Could you check a few things on this drawing? It's one solid part, dimensions in mm from its lowest x, y, z. Round coordinates to 2 decimals unless told otherwise and drop trailing zeros. Loops run counter-clockwise (first coordinate to the right, second up) from the corner with the lowest first, then second, coordinate; pieces in that order, holes last. Notation, with made-up numbers: M -8,14 L 12,14 A13 cw 12,29 Z; hole C -20.75,-32.5 d11. An arc over 180 degrees is marked long. Return JSON: item names as keys, results as strings.
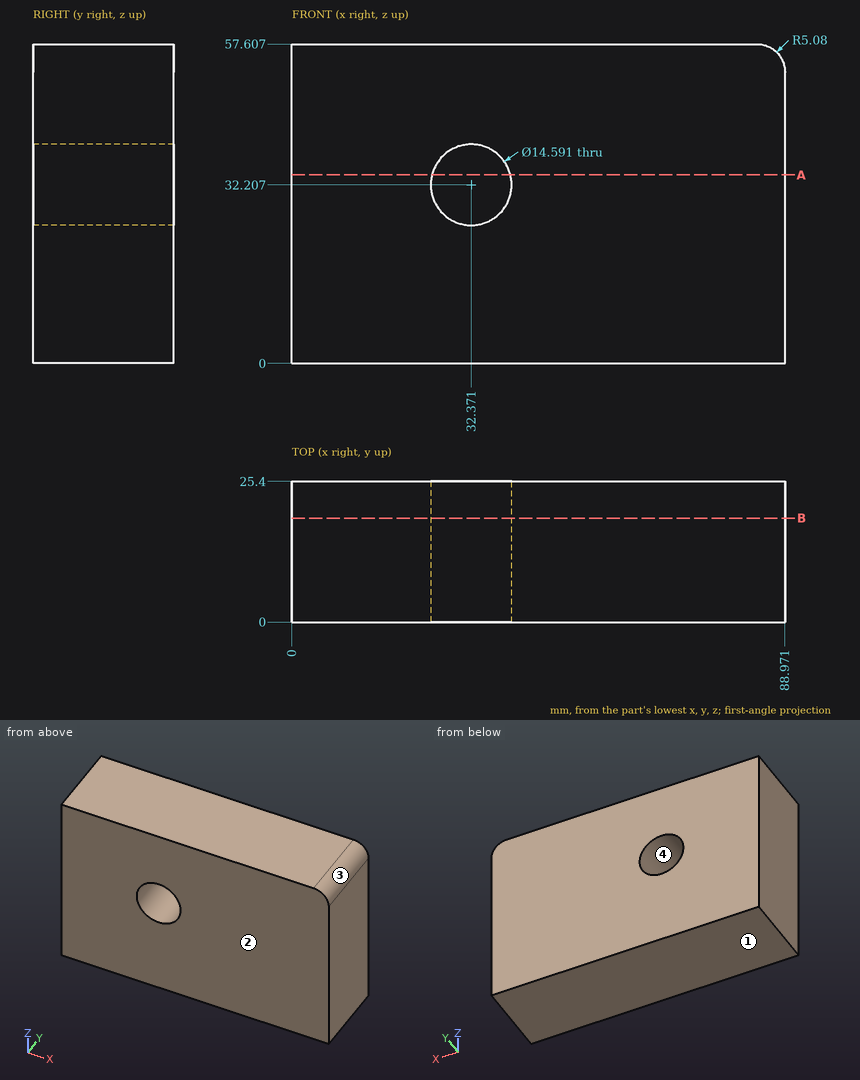
Q1. Thinking about a two-plate mould opening in Z: for the marked faces 1, 2, 3 and 4, which applies, pulls with the +Z half, pulls with the -Z half, needs draft (parallel to the pull), parting line crosses it, or undercut?
Results:
{"face 1": "pulls with the -Z half", "face 2": "needs draft", "face 3": "pulls with the +Z half", "face 4": "undercut"}
Q2. If I drill on line 1 along X through (y, z) = (14, 37.5); line 2 along X through (y, z) = (5.75, 26) (1 decimal); line 3 along Z through (x, y) = (30, 3.75), over which ranges is the centre line in solid material (lowest first)?
Results:
{"line 1": "x = 0 to 27.35, 37.39 to 88.97", "line 2": "x = 0 to 28.5, 36.2 to 89", "line 3": "z = 0 to 25.31, 39.11 to 57.61"}
Q3. Suppose I cut it at B-B, the plane y = 18.75. Please give me the cut outline in (x, z) (1 decimal), plus the area to 3 significant figures.
Results:
{"outline": "M 0,0 L 89,0 L 89,52.5 A5.1 ccw 83.9,57.6 L 0,57.6 Z; hole C 32.4,32.2 d14.6", "area": "4,950 mm2"}
Q4. Suppose I cut it at A-A, the plane z = 34. Please give me the cut outline in (x, y).
Results:
{"outline": "M 0,0 L 25.3,0 L 25.3,25.4 L 0,25.4 Z; M 39.44,0 L 88.97,0 L 88.97,25.4 L 39.44,25.4 Z"}
